Autodesk Fusion 360 part; units mm, degrees
sketch "Sketch1" plane through (0, 0, 0) normal (0, 0, 1) x (1, 0, 0)
  line L0 (0, 0) -> (30, 0)
  line L1 (30, 0) -> (30, 30)
  line L2 (30, 30) -> (0, 30)
  line L3 (0, 30) -> (0, 0)
  circle A0 centre (5, 25) radius 2
  circle A1 centre (25, 25) radius 2
  circle A2 centre (25, 5) radius 2
  circle A3 centre (5, 5) radius 2
  dimension "d1" = 30
  dimension "d2" = 30
  dimension "d3" = 4
  dimension "d4" = 5
  dimension "d5" = 5
  dimension "d6" = 4
  dimension "d7" = 4
  dimension "d8" = 4
  dimension "d9" = 20
  dimension "d10" = 20
  dimension "d11" = 20
  dimension "d12" = 20
  dimension "d13" = 5
  dimension "d14" = 5
extrude "Extrude1" add sketch "Sketch1" along normal blind 5
sketch "Sketch2" plane through (0, 0, 5) normal (0, 0, 1) x (-1, 0, 0)
  circle A0 centre (-5, -5) radius 2
  circle A1 centre (-25, -5) radius 2
  circle A2 centre (-5, -25) radius 2
  circle A3 centre (-25, -25) radius 2
  line L0 (0, -30) -> (0, 0)
  line L1 (0, 0) -> (-30, 0)
  line L2 (-30, 0) -> (-30, -30)
  line L3 (-30, -30) -> (0, -30)
  line L4 (-15, -20) -> (-19, -20)
  line L5 (-19, -20) -> (-19, -10)
  line L6 (-19, -10) -> (-15, -10)
  line L7 (-15, -10) -> (-15, -20)
  dimension "d17" = 4
  dimension "d18" = 10
  dimension "d19" = 15
  dimension "d20" = 10
extrude "Extrude3" add sketch "Sketch2" along normal blind 230 contours L4 L5 L6 L7
Input: part model. Units: mm. Frame: model coordinates. A direction names the side the tool comes from. Give positions to 0.01 mm unless a question says otherwise; leave off trailing zeros. Order: outer loops, then holes, each group sorted by start corner. A loop starts at its lowest first (then second) coordinate and runs counter-clockwise, first axis right, second up. Notation, with made-up numbers: (-34, 77) - (-28, 77) arc R11 ccw to (-28, 98) - close; hole circle Ø8 at (-29, 10.25). An arc over 180 degrees is marked (long way). Write each question's results on one line, items separated by ' | '.
Item 1: Material intervals for line 1 along Y through (x, z) = (5, 2.4); line 2 along Z through (x, y) = (11, 19); line 3 along X through (y, z) = (12.5, 199), sorted ascending.
A:
line 1: y = 0 to 3, 7 to 23, 27 to 30 | line 2: z = 0 to 5 | line 3: x = 15 to 19
Item 2: Access query for faces 1 (the flat face through (17, 10, 118)), 2 (the flat face through (15, 15, 118)), 3 (the flat face through (17, 20, 118)), 4 (the flat face through (19, 15, 118)). Directions: +Z, -Z, +X, -X, +Y, -Y. A direction counts if a zero-diameter tool reaches every point of the face in a straight line with its end or side. Return the directions, or none.
A:
face 1: +Z, +X, -X, -Y | face 2: +Z, -X, +Y, -Y | face 3: +Z, +X, -X, +Y | face 4: +Z, +X, +Y, -Y
Item 3: Draft query along Y for faces 5 (the cylindrical face through (23.4, 26.2, 2.5)), 6 (the flat face through (15, 0, 2)), 7 (the flat face through (15, 30, 2)), 8 (the flat face through (14.8, 15.2, 5)). Return one class per face: released by +Y, released by -Y, zero draft, split by the parting line, or undercut.
A:
face 5: undercut | face 6: released by -Y | face 7: released by +Y | face 8: zero draft
Item 4: Contact query for flat-ended pins moving along their axis: pin 1 Ø3 at (x, y) = (5, 25) entering from -Z; pin 2 Ø2 at (x, z) = (18, 158) entering from -Y; pin 3 Ø5 at (y, z) = (14, 176) entering from +X; pin 4 Ø3 at (x, y) = (24, 19.5) entering from +Z. Output: stop coordinate, or through.
A:
pin 1: passes through | pin 2: stops at y = 10 | pin 3: stops at x = 19 | pin 4: stops at z = 5
Item 5: Section C-C (y = 14.25). Return loops of the section in (x, z).
A:
outline: (0, 0) - (30, 0) - (30, 5) - (19, 5) - (19, 235) - (15, 235) - (15, 5) - (0, 5) - close
Item 6: Section A-A (y = 5). Return loops of the section in (x, z), and give its area (3 significant figures).
A:
outline: (0, 0) - (3, 0) - (3, 5) - (0, 5) - close; (7, 0) - (23, 0) - (23, 5) - (7, 5) - close; (27, 0) - (30, 0) - (30, 5) - (27, 5) - close | area: 110 mm^2
Item 7: Section D-D (z = 127.5). Return loops of the section in (x, y), and give its area (3 significant figures).
A:
outline: (15, 10) - (19, 10) - (19, 20) - (15, 20) - close | area: 40.0 mm^2
